For this review, take the finished solid that the model builds, in its own axes (mm). Face numbers are marked on the shaded views. A direction names the side the tool comes from. Round coordinates to 2 decimals unless told otherwise and drop trailing zeros. Write each loop counter-clockwise with the first axis right and the second up, starting at its lowest first coordinate (ties: lowest second). Pieces come first, ordered by that corner, then holes. Notation, with made-up numbers: M -6,48.25 L 5,48.25 A11 ccw 5,55.25 Z; hole C -39.5,64.5 d4. An arc over 180 degrees is marked long. One line per question, with ' | ' between items.
```python
from build123d import *

# Parameters (mm, degrees)
BOSS_EXTRUDE1_DEPTH       = 50
SKETCH2_OUTSIDE_W         = 128.57
SKETCH2_OUTSIDE_H         = 103.57
SKETCH2_OUTSIDE_R         = 5
SKETCH2_OUTSIDE_R_2       = 3.25
CUT_EXTRUDE34_DEPTH       = 46
CUT_EXTRUDE34_DEPTH_BACK  = 1
BOSS_EXTRUDE3_DEPTH       = 4.5
SUPPORT_DEPTH             = 10
FILLET3_R                 = 2.5
FILLET4_R                 = 7
SKETCH6_R                 = 3.25
LOADCELL_MOUNT_DEPTH      = 1
LOADCELL_MOUNT_DEPTH_BACK = 73.5
WIREHOLE_DEPTH            = 5.18
SKETCH9_R                 = 6.912708826
CUT_EXTRUDE35_DEPTH       = 10


with BuildPart() as part:
    # Sketch1 → Boss-Extrude1 (new body, symmetric)
    with BuildSketch(Plane(origin=(0, 0, 0), x_dir=(0, 0, -1), z_dir=(1, 0, 0))):
        Polygon((0, 0), (0, 45), (4.5, 45), (4.5, 4.5), (75, 4.5), (75, 0), align=None)
    extrude(amount=BOSS_EXTRUDE1_DEPTH, both=True)

    # Sketch2 outside → Cut-Extrude34 (cut, two sides)
    with BuildSketch(Plane(origin=(0, 0, 0), x_dir=(1, 0, 0), z_dir=(0, 1, 0))) as cut_extrude34_sk:
        with Locations((0, 37.5)):
            Rectangle(SKETCH2_OUTSIDE_W, SKETCH2_OUTSIDE_H)
        with BuildLine():
            Line((-40, 30), (-25.836010131, 30))
            ThreePointArc((-25.836010131, 30), (-17.535836731, 26.561955607), (-14.097792338, 18.261782207))
            Line((-14.097792338, 18.261782207), (-14.097792338, 7))
            Line((-14.097792338, 7), (13.661782207, 7))
            Line((13.661782207, 7), (13.661782207, 18.261782207))
            ThreePointArc((13.661782207, 18.261782207), (17.099826599, 26.561955607), (25.4, 30))
            Line((25.4, 30), (40, 30))
            ThreePointArc((40, 30), (47.071067812, 32.928932188), (50, 40))
            Line((50, 40), (50, 65))
            ThreePointArc((50, 65), (47.071067812, 72.071067812), (40, 75))
            Line((40, 75), (-40, 75))
            ThreePointArc((-40, 75), (-47.071067812, 72.071067812), (-50, 65))
            Line((-50, 65), (-50, 40))
            ThreePointArc((-50, 40), (-47.071067812, 32.928932188), (-40, 30))
        make_face(mode=Mode.SUBTRACT)
        with Locations((-25, 52.5)):
            Circle(SKETCH2_OUTSIDE_R)
        with Locations((25, 52.5)):
            Circle(SKETCH2_OUTSIDE_R)
        with Locations((25, 66.04)):
            Circle(SKETCH2_OUTSIDE_R_2)
        with Locations((25, 38.96)):
            Circle(SKETCH2_OUTSIDE_R_2)
        with Locations((34.072580566, 62.550864733)):
            Circle(SKETCH2_OUTSIDE_R_2)
        with Locations((-25, 66.04)):
            Circle(SKETCH2_OUTSIDE_R_2)
        with Locations((-25, 38.96)):
            Circle(SKETCH2_OUTSIDE_R_2)
        with Locations((-34.072580566, 62.550864733)):
            Circle(SKETCH2_OUTSIDE_R_2)
        Polygon((-2.5, 64.24), (2.5, 64.24), (7.5, 59.24), (7.5, 45.76), (2.5, 40.76), (-2.5, 40.76), (-7.5, 45.76), (-7.5, 59.24), align=None)
    extrude(amount=CUT_EXTRUDE34_DEPTH, mode=Mode.SUBTRACT)
    extrude(cut_extrude34_sk.sketch, amount=-CUT_EXTRUDE34_DEPTH_BACK, mode=Mode.SUBTRACT)

    # Sketch4 → Boss-Extrude3 (add)
    with BuildSketch(Plane.XY.offset(-7)):
        with BuildLine():
            Line((-14.097792338, 0), (-14.097792338, 45))
            ThreePointArc((-14.097792338, 45), (-13.365559291, 46.767766953), (-11.597792338, 47.5))
            Line((-11.597792338, 47.5), (13.661782207, 47.5))
            Line((13.661782207, 47.5), (21.222778521, 43.209368433))
            Line((21.222778521, 43.209368433), (21.222778521, 21.944029683))
            Line((21.222778521, 21.944029683), (13.661782207, 17.653398116))
            Line((13.661782207, 17.653398116), (13.661782207, 4.5))
            Line((13.661782207, 4.5), (13.661782207, 0))
            Line((13.661782207, 0), (-14.097792338, 0))
        make_face()
    extrude(amount=BOSS_EXTRUDE3_DEPTH)

    # Sketch → Support (add, symmetric)
    with BuildSketch(Plane(origin=(0, 0, 0), x_dir=(0, 0, -1), z_dir=(1, 0, 0))):
        Polygon((7, 21.944029683), (30, 4.5), (7, 4.5), align=None)
    extrude(amount=SUPPORT_DEPTH, both=True)

    # Fillet3
    fillet3_edges = [part.edges().sort_by_distance(p)[0] for p in [
        (11.830891103, 4.5, -7),
    ]]
    fillet(fillet3_edges, radius=FILLET3_R)

    # Fillet4
    fillet4_edges = [part.edges().sort_by_distance(p)[0] for p in [
        (-0.218005066, 0, -2.5),
    ]]
    fillet(fillet4_edges, radius=FILLET4_R)

    # Sketch6 → LoadCell_Mount (cut, two sides)
    with BuildSketch(Plane.XY.offset(-2.5)) as loadcell_mount_sk:
        with Locations((-0.297792338, 40.083077312)):
            Circle(SKETCH6_R)
        with Locations((-0.297792338, 25.083077312)):
            Circle(SKETCH6_R)
    extrude(amount=LOADCELL_MOUNT_DEPTH, mode=Mode.SUBTRACT)
    extrude(loadcell_mount_sk.sketch, amount=-LOADCELL_MOUNT_DEPTH_BACK, mode=Mode.SUBTRACT)

    # Sketch7 → WireHole (cut)
    with BuildSketch(Plane.XY.offset(-2.5)):
        with BuildLine():
            Line((18.539617084, 41.355633115), (18.539617084, 36.032215871))
            ThreePointArc((18.539617084, 36.032215871), (16.149617084, 33.642215871), (13.759617084, 36.032215871))
            Line((13.759617084, 36.032215871), (13.759617084, 41.355633115))
            ThreePointArc((13.759617084, 41.355633115), (16.149617084, 43.745633115), (18.539617084, 41.355633115))
        make_face()
        with BuildLine():
            Line((18.539617084, 28.355633115), (18.539617084, 23.032215871))
            ThreePointArc((18.539617084, 23.032215871), (16.149617084, 20.642215871), (13.759617084, 23.032215871))
            Line((13.759617084, 23.032215871), (13.759617084, 28.355633115))
            ThreePointArc((13.759617084, 28.355633115), (16.149617084, 30.745633115), (18.539617084, 28.355633115))
        make_face()
    extrude(amount=-WIREHOLE_DEPTH, mode=Mode.SUBTRACT)

    # Sketch9 → Cut-Extrude35 (cut)
    with BuildSketch(Plane(origin=(0, 0, -7), x_dir=(-1, 0, 0), z_dir=(0, 0, -1))):
        with Locations((0, 24.75)):
            Circle(SKETCH9_R)
    extrude(amount=CUT_EXTRUDE35_DEPTH, mode=Mode.SUBTRACT)


solid = part.part
```
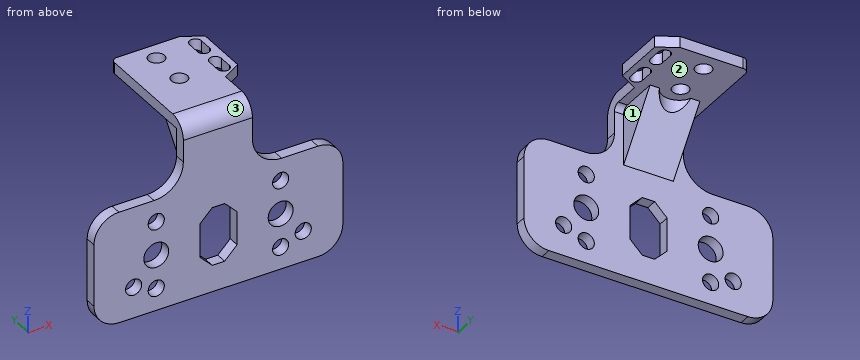
Item 1: Take a section at A-A (z = -52.5). Write out the cut boundary in (x, y).
Results:
outline: M -50,0 L -30,0 L -30,4.5 L -50,4.5 Z; M -20,0 L -7.5,0 L -7.5,4.5 L -20,4.5 Z; M 7.5,0 L 20,0 L 20,4.5 L 7.5,4.5 Z; M 30,0 L 50,0 L 50,4.5 L 30,4.5 Z
Item 2: To check wall thickness, follow line 1 along Z through (x, y) = (25, 3); line 2 along X through (y, z) = (1.6, -66.04); line 3 along Y through (x, z) = (30, -66). State the ranges of each line that lie inside material, in increasing order. Write a range as from..to.
Results:
line 1: -75..-69.29, -62.79..-57.5, -47.5..-42.21, -35.71..-29.99 | line 2: -49.95..-28.25, -21.75..21.75, 28.25..49.95 | line 3: 0..4.5
Item 3: Take a section at D-D (y = 3). State how many separate pieces and enclosed holes the cut face has, then the cut area to 3 significant figures.
Results:
separate pieces: 1 | enclosed holes: 9 | area: 4,540 mm2
Item 4: Insertion check: pin 1 Ø12.5 at (y, z) = (10, -11.5) entering from +X; pin 2 Ø5 at (x, y) = (-19, 34) entering from -Z; pin 3 Ø5 at (y, z) = (27, -5) entering from -X; pin 4 Ø1.3 at (y, z) = (30, -3.5) entering from +X. Each pin has a flat end and moves straight along its axis. Give the tip position at first contact, or say it passes through.
Results:
pin 1: x = 13.66 | pin 2: through | pin 3: x = -14.1 | pin 4: x = 21.22
Item 5: Take a section at C-C (z = -22). Write out the cut boundary in (x, y).
Results:
outline: M -14.71,0 L 14.27,0 L 14.27,4.5 L 10,4.5 L 10,10.57 L -10,10.57 L -10,4.5 L -14.71,4.5 Z
Item 6: Machinability: for the marked faces 1, 2 and 3, which of the approach directions +Z, -Z, +X, -X, +Y, -Y give a long, thin tool a straight path to every point of the face, cutting with its end or side? Answer none if there is none.
Results:
face 1: -Z, +X, +Y | face 2: -Z, +Y | face 3: +Z, +X, -X, -Y
Item 7: Take a section at B-B (y = 38.5). Write out the cut boundary in (x, z).
Results:
outline: M -14.1,-7 L -3.14,-7 L -3.14,-2.5 L -14.1,-2.5 Z; M 2.54,-7 L 13.76,-7 L 13.76,-2.5 L 2.54,-2.5 Z; M 18.54,-7 L 21.22,-7 L 21.22,-2.5 L 18.54,-2.5 Z
